Build history of the part. All positions in model axes, mm. Round coordinates to 2 decimals unless told otherwise and drop trailing zeros. One line per item, written item: value. Start each with the question number.
Item 1: Pin check, flat tips, straight feed: pin 1 (0.7 mm diameter, centred on x = 29.5, y = 5, fed in from -Z); pin 2 (3.5 mm diameter, centred on x = 3, y = 12, fed in from -Z); pin 3 (0.7 mm diameter, centred on y = 6.5, z = 7, fed in from -X). Stop position of each tip, or through.
Item 2: Band-saw the part on B-B, the plane y = 80.8. Give the number of separate pieces and of enclosed holes in the cut face, then the cut area to 3 significant figures.
Item 3: Probe L1, parallel to X at y = 80.8, z = 2; L2, parallel to X at y = 8, z = 1.5; L3, parallel to Y at x = 55, z = 2.25. List the from-to ranges inside material, lowest first.
```python
from build123d import *

# Parameters (mm, degrees)
SKIZZE1_W                        = 67
SKIZZE1_H                        = 95
AUFSATZ_LINEAR_AUSTRAGEN1_DEPTH  = 8
SKIZZE2_W                        = 56.7
SKIZZE2_H                        = 85.1
SCHNITT_LINEAR_AUSTRAGEN1_DEPTH  = 0.5
SCHNITT_LINEAR_START             = -7.5
SKIZZE3_W                        = 49.96
SKIZZE3_H                        = 74.44
SCHNITT_LINEAR_AUSTRAGEN2_DEPTH  = 7.5
SCHNITT_LINEAR_AUSTRAGEN3_REACH  = 9.5
SKIZZE4_W                        = 16
SKIZZE4_H                        = 2
SKIZZE5_W                        = 56.8
SKIZZE5_H                        = 85.3
SCHNITT_LINEAR_AUSTRAGEN4_DEPTH  = 6.9
FASE1_SIZE                       = 2
FASE2_SIZE                       = 0.5
SKIZZE8_W                        = 56.8
SKIZZE8_H                        = 3
SCHNITT_LINEAR_AUSTRAGEN5_DEPTH  = 2
SKIZZE10_W                       = 56.8
SKIZZE10_H                       = 1.5
AUFSATZ_LINEAR_AUSTRAGEN2_DEPTH  = 85.3
SCHNITT_LINEAR_AUSTRAGEN6_REACH  = 7.6
SKIZZE12_W                       = 56.8
SKIZZE12_H                       = 82.3
VERRUNDUNG2_R                    = 2
FASE3_SIZE                       = 3
FASE3_SIZE2                      = 0.803847577
SCHNITT_LINEAR_AUSTRAGEN9_DEPTH  = 3
FASE8_SIZE                       = 0.3
SKIZZE18_W                       = 1.65
SKIZZE18_H                       = 4.4
SCHNITT_LINEAR_AUSTRAGEN10_DEPTH = 4.1
AUFSATZ_LINEAR_START             = 1.65
SKIZZE20_R                       = 1.75
AUFSATZ_LINEAR_AUSTRAGEN7_DEPTH  = 4
SCHNITT_LINEAR_START_2           = -1
SKIZZE21_R                       = 1.05
SCHNITT_LINEAR_AUSTRAGEN12_DEPTH = 6.65
LINEARES_MUSTER1_COUNT           = 2
LINEARES_MUSTER1_PITCH           = 68.8
LINEARES_START                   = 1.65
LINEARES_MUSTER1_COPY_1_SKETCH_R = 1.75
LINEARES_MUSTER1_COPY_1_DEPTH    = 4
LINEARES_START_2                 = -1
LINEARES_MUSTER1_COPY_2_SKETCH_R = 1.05
LINEARES_MUSTER1_COPY_2_DEPTH    = 6.65
LINEARES_MUSTER1_COPY_3_SKETCH_W = 1.65
LINEARES_MUSTER1_COPY_3_SKETCH_H = 4.4
LINEARES_MUSTER1_COPY_3_DEPTH    = 4.1


with BuildPart() as part:
    # Skizze1 → Aufsatz-Linear austragen1 (new body)
    with BuildSketch(Plane.XY):
        with Locations((33.5, 47.5)):
            Rectangle(SKIZZE1_W, SKIZZE1_H)
    extrude(amount=AUFSATZ_LINEAR_AUSTRAGEN1_DEPTH)

    # Skizze2 → Schnitt-Linear austragen1 (cut)
    with BuildSketch(Plane.XY.offset(8)):
        with Locations((33.5, 47.5)):
            Rectangle(SKIZZE2_W, SKIZZE2_H)
    extrude(amount=-SCHNITT_LINEAR_AUSTRAGEN1_DEPTH, mode=Mode.SUBTRACT)

    # Skizze3 → Schnitt-Linear austragen2 (cut)
    with BuildSketch(Plane.XY.offset(7.5).offset(SCHNITT_LINEAR_START)):
        with Locations((33.5, 49.57)):
            Rectangle(SKIZZE3_W, SKIZZE3_H)
    extrude(amount=SCHNITT_LINEAR_AUSTRAGEN2_DEPTH, mode=Mode.SUBTRACT)

    # Skizze4 → Schnitt-Linear austragen3 (cut, up to next)
    with BuildSketch(Plane.XY.offset(7.5), mode=Mode.PRIVATE) as schnitt_linear_austragen3_sk1:
        with Locations((20.15, 6.45)):
            Rectangle(SKIZZE4_W, SKIZZE4_H)
    schnitt_linear_austragen3_tool1 = extrude(schnitt_linear_austragen3_sk1.sketch, amount=-SCHNITT_LINEAR_AUSTRAGEN3_REACH, mode=Mode.PRIVATE) & part.part
    add(schnitt_linear_austragen3_tool1.solids().sort_by_distance((20.15, 6.45, 7.5))[0], mode=Mode.SUBTRACT)

    # Skizze5 → Schnitt-Linear austragen4 (cut)
    with BuildSketch(Plane(origin=(0, 0, 0), x_dir=(-1, 0, 0), z_dir=(0, 0, -1))):
        with Locations((-33.5, 47.5)):
            Rectangle(SKIZZE5_W, SKIZZE5_H)
    extrude(amount=-SCHNITT_LINEAR_AUSTRAGEN4_DEPTH, mode=Mode.SUBTRACT)

    # Fase1
    fase1_edges = [part.edges().sort_by_distance(p)[0] for p in [
        (67, 47.5, 8),
        (33.5, 95, 8),
        (0, 47.5, 8),
        (33.5, 0, 8),
    ]]
    chamfer(fase1_edges, length=FASE1_SIZE)

    # Fase2
    fase2_edges = [part.edges().sort_by_distance(p)[0] for p in [
        (20.15, 5.45, 6.9),
    ]]
    chamfer(fase2_edges, length=FASE2_SIZE)

    # Skizze8 → Schnitt-Linear austragen5 (cut)
    with BuildSketch(Plane.XZ.offset(-90.15)):
        with Locations((33.5, 5.4)):
            Rectangle(SKIZZE8_W, SKIZZE8_H)
    extrude(amount=-SCHNITT_LINEAR_AUSTRAGEN5_DEPTH, mode=Mode.SUBTRACT)

    # Skizze10 → Aufsatz-Linear austragen2 (add)
    with BuildSketch(Plane.XZ.offset(-90.15)):
        with Locations((33.5, 3.15)):
            Rectangle(SKIZZE10_W, SKIZZE10_H)
    extrude(amount=AUFSATZ_LINEAR_AUSTRAGEN2_DEPTH)

    # Skizze12 → Schnitt-Linear austragen6 (cut, up to next)
    with BuildSketch(Plane(origin=(0, 0, 2.4), x_dir=(-1, 0, 0), z_dir=(0, 0, -1)), mode=Mode.PRIVATE) as schnitt_linear_austragen6_sk1:
        with Locations((-33.5, 47.5)):
            Rectangle(SKIZZE12_W, SKIZZE12_H)
    schnitt_linear_austragen6_tool1 = extrude(schnitt_linear_austragen6_sk1.sketch, amount=-SCHNITT_LINEAR_AUSTRAGEN6_REACH, mode=Mode.PRIVATE) & part.part
    add(schnitt_linear_austragen6_tool1.solids().sort_by_distance((33.5, 47.5, 2.4))[0], mode=Mode.SUBTRACT)

    # Verrundung2
    verrundung2_edges = [part.edges().sort_by_distance(p)[0] for p in [
        (0, 0, 3),
        (0, 95, 3),
        (67, 0, 3),
        (67, 95, 3),
    ]]
    fillet(verrundung2_edges, radius=VERRUNDUNG2_R)

    # Fase3
    fase3_edges = [part.edges().sort_by_distance(p)[0] for p in [
        (33.5, 88.65, 3.9),
    ]]
    fase3_side = [part.faces().sort_by_distance(p)[0] for p in [
        (33.5, 90.4, 3.9),
    ]]
    chamfer(fase3_edges, length=FASE3_SIZE, length2=FASE3_SIZE2, reference=fase3_side[0])

    # Skizze14 → Schnitt-Linear austragen9 (cut)
    with BuildSketch(Plane(origin=(0, 0, 0), x_dir=(-1, 0, 0), z_dir=(0, 0, -1))):
        with BuildLine():
            Line((-64, 94), (-3, 94))
            ThreePointArc((-3, 94), (-1.585786438, 93.414213562), (-1, 92))
            Line((-1, 92), (-1, 3))
            ThreePointArc((-1, 3), (-1.585786438, 1.585786438), (-3, 1))
            Line((-3, 1), (-64, 1))
            ThreePointArc((-64, 1), (-65.414213562, 1.585786438), (-66, 3))
            Line((-66, 3), (-66, 92))
            ThreePointArc((-66, 92), (-65.414213562, 93.414213562), (-64, 94))
        make_face()
        with BuildLine():
            ThreePointArc((-64.8, 4.2), (-64.214213562, 2.785786438), (-62.8, 2.2))
            Line((-62.8, 2.2), (-4.2, 2.2))
            ThreePointArc((-4.2, 2.2), (-2.785786438, 2.785786438), (-2.2, 4.2))
            Line((-2.2, 4.2), (-2.2, 90.8))
            ThreePointArc((-2.2, 90.8), (-2.785786438, 92.214213562), (-4.2, 92.8))
            Line((-4.2, 92.8), (-62.8, 92.8))
            ThreePointArc((-62.8, 92.8), (-64.214213562, 92.214213562), (-64.8, 90.8))
            Line((-64.8, 90.8), (-64.8, 4.2))
        make_face(mode=Mode.SUBTRACT)
    extrude(amount=-SCHNITT_LINEAR_AUSTRAGEN9_DEPTH, mode=Mode.SUBTRACT)

    # Fase8
    fase8_edges = [part.edges().sort_by_distance(p)[0] for p in [
        (64.214213562, 2.785786438, 0),
        (33.5, 2.2, 0),
        (2.2, 47.5, 0),
        (2.785786438, 92.214213562, 0),
        (64.214213562, 92.214213562, 0),
        (64.8, 47.5, 0),
        (33.5, 92.8, 0),
        (2.785786438, 2.785786438, 0),
        (61.9, 47.5, 0),
        (33.5, 4.85, 0),
        (5.1, 47.5, 0),
        (33.5, 90.15, 0),
    ]]
    chamfer(fase8_edges, length=FASE8_SIZE)

    # Skizze18 → Schnitt-Linear austragen10 (cut)
    with BuildSketch(Plane(origin=(5.1, 0, 0), x_dir=(0, 0, -1), z_dir=(1, 0, 0))):
        with Locations((-4.825, 80.8)):
            Rectangle(SKIZZE18_W, SKIZZE18_H)
    schnitt_linear_austragen10 = extrude(amount=-SCHNITT_LINEAR_AUSTRAGEN10_DEPTH, mode=Mode.SUBTRACT)

    # Spiegeln6: Schnitt-Linear austragen10 across plane
    add(schnitt_linear_austragen10.mirror(Plane.ZY.offset(-33.5)), mode=Mode.SUBTRACT)

    # Skizze20 → Aufsatz-Linear austragen7 (add)
    with BuildSketch(Plane(origin=(0, 0, 5.65), x_dir=(-1, 0, 0), z_dir=(0, 0, -1)).offset(AUFSATZ_LINEAR_START)):
        with Locations((-3, 80.8)):
            Circle(SKIZZE20_R)
    aufsatz_linear_austragen7 = extrude(amount=AUFSATZ_LINEAR_AUSTRAGEN7_DEPTH)

    # Skizze21 → Schnitt-Linear austragen12 (cut)
    with BuildSketch(Plane(origin=(0, 0, 5.65), x_dir=(-1, 0, 0), z_dir=(0, 0, -1)).offset(SCHNITT_LINEAR_START_2)):
        with Locations((-3, 80.8)):
            Circle(SKIZZE21_R)
    schnitt_linear_austragen12 = extrude(amount=SCHNITT_LINEAR_AUSTRAGEN12_DEPTH, mode=Mode.SUBTRACT)

    # Spiegeln1: Aufsatz-Linear austragen7, Schnitt-Linear austragen12 across plane
    add(aufsatz_linear_austragen7.mirror(Plane.ZY.offset(-33.5)))
    add(schnitt_linear_austragen12.mirror(Plane.ZY.offset(-33.5)), mode=Mode.SUBTRACT)

    # Lineares Muster1: Schnitt-Linear austragen10, Aufsatz-Linear austragen7, Schnitt-Linear austragen12 ×2
    with Locations(*[(0, -i * LINEARES_MUSTER1_PITCH, 0) for i in range(1, LINEARES_MUSTER1_COUNT)]):
        add(schnitt_linear_austragen10, mode=Mode.SUBTRACT)
        add(aufsatz_linear_austragen7)
        add(schnitt_linear_austragen12, mode=Mode.SUBTRACT)

    # Lineares Muster1 copy 1 sketch → Lineares Muster1 copy 1 (add)
    with BuildSketch(Plane(origin=(67, -68.8, 5.65), x_dir=(1, 0, 0), z_dir=(0, 0, -1)).offset(LINEARES_START)):
        with Locations((-3, -80.8)):
            Circle(LINEARES_MUSTER1_COPY_1_SKETCH_R)
    extrude(amount=LINEARES_MUSTER1_COPY_1_DEPTH)

    # Lineares Muster1 copy 2 sketch → Lineares Muster1 copy 2 (cut)
    with BuildSketch(Plane(origin=(67, -68.8, 5.65), x_dir=(1, 0, 0), z_dir=(0, 0, -1)).offset(LINEARES_START_2)):
        with Locations((-3, -80.8)):
            Circle(LINEARES_MUSTER1_COPY_2_SKETCH_R)
    extrude(amount=LINEARES_MUSTER1_COPY_2_DEPTH, mode=Mode.SUBTRACT)

    # Lineares Muster1 copy 3 sketch → Lineares Muster1 copy 3 (cut)
    with BuildSketch(Plane(origin=(61.9, -68.8, 0), x_dir=(0, 0, -1), z_dir=(-1, 0, 0))):
        with Locations((-4.825, -80.8)):
            Rectangle(LINEARES_MUSTER1_COPY_3_SKETCH_W, LINEARES_MUSTER1_COPY_3_SKETCH_H)
    extrude(amount=-LINEARES_MUSTER1_COPY_3_DEPTH, mode=Mode.SUBTRACT)


solid = part.part
```
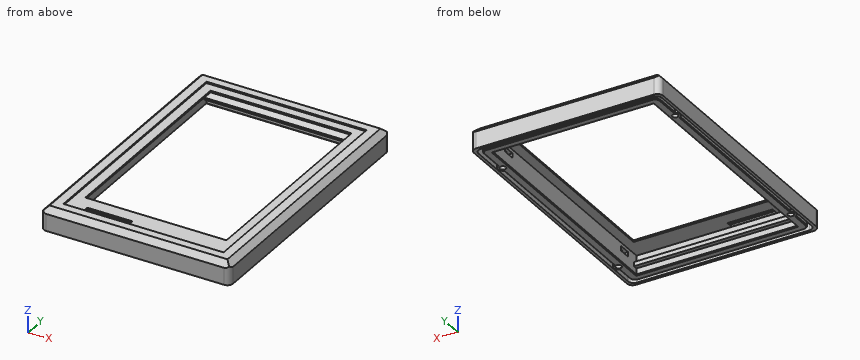
Output:
1. pin 1: stops at z = 0.1
1. pin 2: stops at z = 0
1. pin 3: stops at x = 0.65
2. separate pieces: 4
2. enclosed holes: 0
2. area: 45.6 mm²
3. L1: x = 0 to 1, 1.25 to 1.95, 4.05 to 5.1, 61.9 to 62.95, 65.05 to 65.75, 66 to 67
3. L2: x = 0 to 1, 2.2 to 5.1, 61.9 to 64.8, 66 to 67
3. L3: y = 0 to 1, 2.2 to 4.85, 90.15 to 92.8, 94 to 95
